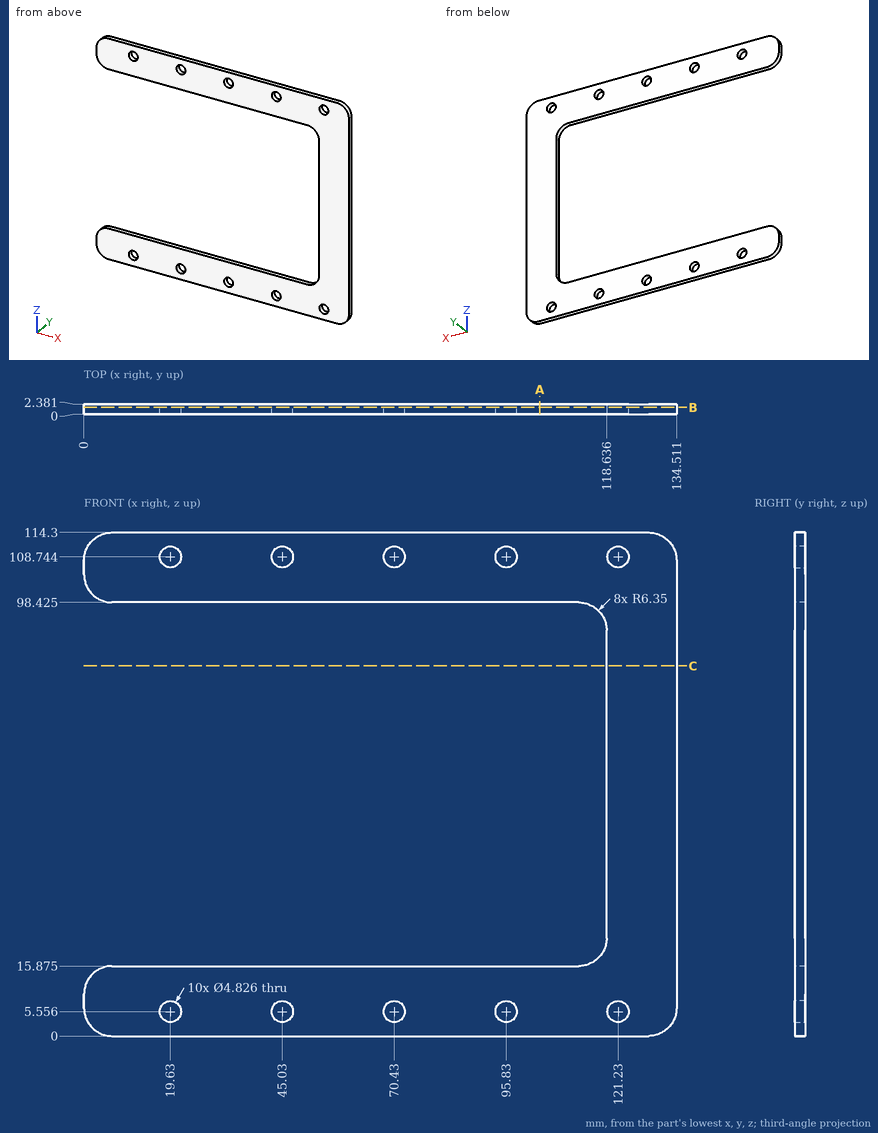
Verification items for this drawing (mm, ordinates from the low corner). Give positions to 0.01 mm unless a question says otherwise; leave off trailing zeros. Loops run counter-clockwise (first coordinate to the right, second up) from the corner with the lowest first, then second, coordinate; pieces in that order, holes last. Notation, with made-up numbers: (20.25, 29) - (36.25, 29) arc R20 cw to (36.25, 61) - close; hole circle Ø3 at (23, -8). An arc over 180 degrees is marked (long way). Write item = value, one per line. Start each with the question number.
Q1. Thickness scan on line 1 (Z direction, x = 82, y = 0.55) (1 decimal); line 2 (Z direction, x = 72, y = 1.85) (1 decimal); line 3 (Z direction, x = 21.5, y = 2.35) (1 decimal). Record the ranges inside material, lowest first.
Q2. Cross-section at B-B, the plane y = 1.6. State how many separate pieces and enclosed holes the cut face has, and give its area (3 significant figures).
Q3. Cross-section at C-C, the plane z = 84. Enter the section's corners in (x, y) (1 decimal), and give its area (3 significant figures).
Q4. Depth check by flat-ended pin: P1, Ø6, axis at x = 28.5, z = 96, coming from the +Y side. Enter the tip coordinate at first touch or a pass-through.
Q5. Cross-section at A-A, the plane x = 103.5. Enter the section's corners in (y, z) (1 decimal).
Answer key:
q1.line_1 = 0 to 15.9, 98.4 to 114.3
q1.line_2 = 0 to 3.7, 7.4 to 15.9, 98.4 to 106.9, 110.6 to 114.3
q1.line_3 = 0 to 4, 7.1 to 15.9, 98.4 to 107.2, 110.3 to 114.3
q2.separate_pieces = 1
q2.enclosed_holes = 10
q2.area = 5,360 mm^2
q3.outline = (118.6, 0) - (134.5, 0) - (134.5, 2.4) - (118.6, 2.4) - close
q3.area = 37.8 mm^2
q4.P1 = 2.38
q5.outline = (0, 0) - (2.4, 0) - (2.4, 15.9) - (0, 15.9) - close; (0, 98.4) - (2.4, 98.4) - (2.4, 114.3) - (0, 114.3) - close
